Read the model definition and answer for the solid it produces. Units are mm, in the model's axes. A direction names the side the tool comes from. Coordinates: 2 decimals unless noted, no trailing zeros. Write each loop counter-clockwise with the first axis right and the second up, starting at its lowest first coordinate (ties: lowest second). Pieces come first, ordered by that corner, then holes. Notation, with made-up numbers: (18, 36.5) -> (29, 36.5) arc R20 cw to (29, 58.5) -> close; hole circle Ø3 at (-16.5, -20.5). An arc over 180 degrees is marked (long way). Return JSON: item names as keys, results as strings.
from build123d import *

# Parameters (mm, degrees)
F0_R     = 2
F1_DEPTH = 8
F2_R     = 2
F3_DEPTH = 60
F4_R     = 3.99999
F5_R     = 1.5
F6_R     = 3.75
F7_DEPTH = 6
F8_SIZE  = 1
F9_R     = 1.5


# Not quite as in the source:
# - a fillet or chamfer is up to 0.001 mm smaller than in the source, because OpenCascade refuses the exact size


with BuildPart() as f1:
    # F0 (on Top) → F1 (new body)
    with BuildSketch(Plane.XY):
        Polygon((25, -15), (25, 15), (12.5, 15), (12.5, 5), (-12.5, 5), (-12.5, 15), (-25, 15), (-25, -15), align=None)
        with Locations((-15, -6.3565024175)):
            Circle(F0_R, mode=Mode.SUBTRACT)
        with Locations((0, -6.3565024175)):
            Circle(F0_R, mode=Mode.SUBTRACT)
        with Locations((15, -6.3565024175)):
            Circle(F0_R, mode=Mode.SUBTRACT)
    extrude(amount=F1_DEPTH)

    # F2 (on face) → F3 (cut)
    with BuildSketch(Plane(origin=(-25, 0, 0), x_dir=(0, -1, 0), z_dir=(-1, 0, 0))):
        with Locations((-10.8748758212, 4)):
            Circle(F2_R)
    extrude(amount=-F3_DEPTH, mode=Mode.SUBTRACT)

    # F4 (radius 4 in the source; OpenCascade refuses exactly that, so slightly less here)
    f4_edges = [f1.edges().sort_by_distance(p)[0] for p in [
        (-18.75, 15, 8),
        (18.75, 15, 8),
        (-18.75, 15, 0),
        (18.75, 15, 0),
    ]]
    fillet(f4_edges, radius=F4_R)

    # F5
    f5_edges = [f1.edges().sort_by_distance(p)[0] for p in [
        (0, 5, 8),
        (0, -15, 8),
    ]]
    fillet(f5_edges, radius=F5_R)

    # F6 (on face) → F7 (cut)
    with BuildSketch(Plane.XY.offset(8)):
        with Locations((-15, -6.3565024175)):
            Circle(F6_R)
        with Locations((0, -6.3565024175)):
            Circle(F6_R)
        with Locations((15, -6.3565024175)):
            Circle(F6_R)
    extrude(amount=-F7_DEPTH, mode=Mode.SUBTRACT)

    # F8
    f8_edges = [f1.edges().sort_by_distance(p)[0] for p in [
        (-17, -6.356502, 2),
        (-2, -6.356502, 2),
        (13, -6.356502, 2),
    ]]
    chamfer(f8_edges, length=F8_SIZE)

    # F9
    f9_edges = [f1.edges().sort_by_distance(p)[0] for p in [
        (25, -1.249995, 8),
        (-25, -1.249995, 8),
    ]]
    fillet(f9_edges, radius=F9_R)


solid = f1.part
1. Consider L1, parallel to X at y = 7, z = 5.5; L2, parallel to X at y = -6.75, z = 5; L3, parallel to Z at x = -13, y = 12.5. Determine where each line is inside the solid, lowest interval first.
Taken from the geometry:
{"L1": "x = -25 to -12.5, 12.5 to 25", "L2": "x = -25 to -18.73, -11.27 to -3.73, 3.73 to 11.27, 18.73 to 25", "L3": "z = 0.29 to 2.83, 5.17 to 7.71"}
2. The part is cut by section A-A (x = -15). Count the separate pieces of the cut face and the enclosed holes in it, then the cut area to 3 significant figures.
Taken from the geometry:
{"separate pieces": "2", "enclosed holes": "1", "area": "166 mm2"}
3. Flat-ended cylindrical pins translate along their axes: pin 1 Ø2 at (x, y) = (-14, -7.5) entering from +Z; pin 2 Ø4 at (x, y) = (16, -7) entering from +Z; pin 3 Ø8 at (x, y) = (6, 11) entering from -Z. Find the tip coordinate at first contact, or state that the pin passes through.
Taken from the geometry:
{"pin 1": "stops at z = 1.52", "pin 2": "stops at z = 2", "pin 3": "passes through"}
4. A tool of negligible diameter and unlimited length cuts with its end or side. For faces 1 (the face through (24.57, -14.55, 3.3)), 2 (the face through (0, -3, 2)), from which of +Z, -Z, +X, -X, +Y, -Y can it reach the whole face along a straight path? Write none if from no direction.
Taken from the geometry:
{"face 1": "+Z, -Z, +X, -Y", "face 2": "+Z"}
5. For a pull along X with two mould halves and no side action, classify faces 3 (the face through (12.5, 8, 4)), 4 (the face through (15, -3, 2)), 5 (the face through (24.57, -1.08, 7.55)), 6 (the face through (0, -15, 3)) as +X half, -X half, draft (parallel to the pull), parting line (faces both ways), or undercut.
Taken from the geometry:
{"face 3": "undercut", "face 4": "undercut", "face 5": "+X half", "face 6": "draft"}
6. The part is cut by section B-B (x = 0). Determine the outline of the cut face in (y, z).
Taken from the geometry:
{"outline": "(-15, 0) -> (-8.36, 0) -> (-8.36, 1) -> (-9.36, 2) -> (-10.11, 2) -> (-10.11, 8) -> (-13.5, 8) arc R1.5 ccw to (-15, 6.5) -> close; (-4.36, 0) -> (5, 0) -> (5, 6.5) arc R1.5 ccw to (3.5, 8) -> (-2.61, 8) -> (-2.61, 2) -> (-3.36, 2) -> (-4.36, 1) -> close"}
